The listing builds one solid part. Answer for the finished solid, in the listing's coordinates (mm). A direction names the side the tool comes from. Give positions to 0.01 mm unless a question says otherwise; leave off trailing zeros. Write each loop counter-clockwise with the first axis right and the second up, starting at its lowest first coordinate (ties: lowest second). Pieces come first, ordered by that corner, then holes. Notation, with made-up numbers: (-3, -7) - (3, -7) arc R38 ccw to (3, 31) - close; hole circle Ø7 at (-23, 29.25). An arc over 180 degrees is marked (long way). Return JSON: item names as keys, results as strings.
from build123d import *

# Parameters (mm, degrees)
F0_R      = 40
F1_DEPTH  = 20
F3_DEPTH  = 25
F4_R      = 3
F5_DEPTH  = 17.5
F7_R      = 5.5
F8_DEPTH  = 25
F9_R      = 3
F10_DEPTH = 15


with BuildPart() as f1:
    # F0 (on Front) → F1 (new body)
    with BuildSketch(Plane.XZ):
        with BuildLine():
            Line((0, 20), (0, 0))
            Line((0, 0), (160, 0))
            Line((160, 0), (160, 20))
            Line((160, 20), (135.8997487421, 81.7994974843))
            ThreePointArc((135.8997487421, 81.7994974843), (80, 120), (24.1002512579, 81.7994974843))
            Line((24.1002512579, 81.7994974843), (0, 20))
        make_face()
        with Locations((80, 60)):
            Circle(F0_R, mode=Mode.SUBTRACT)
    extrude(amount=F1_DEPTH)

    # F2 (on face) → F3 (cut)
    with BuildSketch(Plane.XZ.offset(20)):
        Polygon((118.0051983823, 117.4108353592), (118.0051983823, 60), (120, 60), (120, 117.2667294741), align=None)
    extrude(amount=-F3_DEPTH, mode=Mode.SUBTRACT)

    # F4 (on face) → F5 (cut, symmetric)
    with BuildSketch(Plane.YZ.offset(118.0051983823)):
        with Locations((-10, 91.4284922857)):
            Circle(F4_R)
    extrude(amount=F5_DEPTH, both=True, mode=Mode.SUBTRACT)

    # F7 (on offset) → F8 (cut)
    with BuildSketch(Plane(origin=(125, 0, 0), x_dir=(0, -1, 0), z_dir=(-1, 0, 0))):
        with Locations((10, 91.4284922857)):
            Circle(F7_R)
    extrude(amount=-F8_DEPTH, mode=Mode.SUBTRACT)

    # F9 (on face) → F10 (cut)
    with BuildSketch(Plane(origin=(0, 0, 0), x_dir=(1, 0, 0), z_dir=(0, 0, -1))):
        with Locations((20, 10)):
            Circle(F9_R)
        with Locations((140, 10)):
            Circle(F9_R)
        with Locations((80, 10)):
            Circle(F9_R)
    extrude(amount=-F10_DEPTH, mode=Mode.SUBTRACT)


solid = f1.part
Item 1: A cutting plane is placed at D-D on x = 123. Determine the outline of the cut face in (y, z).
Answer below:
{"outline": "(-20, 0) - (0, 0) - (0, 101.84) - (-20, 101.84) - close; hole circle Ø6 at (-10, 91.43)"}
Item 2: Consider L1, parallel to X at y = -10, z = 5; L2, parallel to Z at x = 80, y = -15.5; L3, parallel to X at y = -14.25, z = 84.5. Determine where each line is inside the solid, lowest interval first.
Answer below:
{"L1": "x = 0 to 17, 23 to 77, 83 to 137, 143 to 160", "L2": "z = 0 to 20, 100 to 120", "L3": "x = 25.23 to 48.38, 111.62 to 118.01, 120 to 134.77"}
Item 3: A cutting plane is placed at C-C on z = 10.5. Determine the outline of the cut face in (x, y).
Answer below:
{"outline": "(0, -20) - (160, -20) - (160, 0) - (0, 0) - close; hole circle Ø6 at (20, -10); hole circle Ø6 at (80, -10); hole circle Ø6 at (140, -10)"}
Item 4: A cutting plane is placed at A-A on x = 80. Determine the outline of the cut face in (y, z), then the cut area to 3 significant figures.
Answer below:
{"outline": "(-20, 0) - (-13, 0) - (-13, 15) - (-7, 15) - (-7, 0) - (0, 0) - (0, 20) - (-20, 20) - close; (-20, 100) - (0, 100) - (0, 120) - (-20, 120) - close", "area": "710 mm²"}
Item 5: A cutting plane is placed at B-B on z = 47. Determine the outline of the cut face in (x, y).
Answer below:
{"outline": "(10.53, -20) - (42.17, -20) - (42.17, 0) - (10.53, 0) - close; (117.83, -20) - (149.47, -20) - (149.47, 0) - (117.83, 0) - close"}
Item 6: For faces 4 (the face through (111.3, -10.4, 94.4)), 5 (the face through (80, -10, 15)), 6 (the face through (12.22, -9.86, 51.33)), 7 (the face through (148.119, -9.86, 50.467)), 8 (the face through (118.005, -10, 86)), determine the directions among +Z, -Z, +X, -X, +Y, -Y from which every point of the face is accessible in a straight line to the end or side of a thin tool.
Answer below:
{"face 4": "+X", "face 5": "-Z", "face 6": "+Z, -X, +Y, -Y", "face 7": "+Z, +X, +Y, -Y", "face 8": "+Z, +Y, -Y"}
Item 7: The mould has two halves that part along X. Classify faces 1 (the face through (65.545, -9.86, 118.233)), 2 (the face through (97, 0, 21)), 3 (the face through (142.86, -10.9, 7.4)): +X half, -X half, draft (parallel to the pull), parting line (faces both ways), or undercut.
Answer below:
{"face 1": "parting line", "face 2": "draft", "face 3": "undercut"}
Item 8: Flat-ended cylindrical pins translate along their axes: P1, Ø7, axis at y = -10, z = 91.43, coming from the +X side; P2, Ø2, axis at y = -13, z = 85, coming from the -X side; P3, Ø1, axis at y = -4, z = 28.5, coming from the -X side. Find the tip coordinate at first contact, or state that the pin passes through.
Answer below:
{"P1": "stops at x = 125", "P2": "stops at x = 25.01", "P3": "stops at x = 3.12"}
